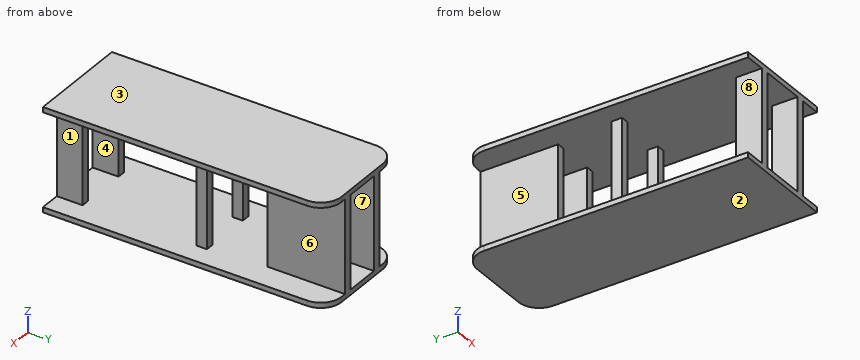
```python
from build123d import *

# Parameters (mm, degrees)
SKETCH_1_W      = 200
SKETCH_1_H      = 550
EXTRUDE_2_DEPTH = 10
FILLET_2_R      = 40
SKETCH_2_W      = 16
SKETCH_2_H      = 50
SKETCH_2_H_2    = 20
SKETCH_2_H_3    = 150
EXTRUDE_4_DEPTH = 90
SKETCH_3_W      = 200
SKETCH_3_H      = 550
EXTRUDE_5_DEPTH = 10
FILLET_5_R      = 40


with BuildPart() as part:
    # 스케치1 → 보스-돌출2 (new body)
    with BuildSketch(Plane.XY):
        with Locations((100, 275)):
            Rectangle(SKETCH_1_W, SKETCH_1_H)
    extrude(amount=EXTRUDE_2_DEPTH)

    # 필렛2
    fillet_2_edges = [part.edges().sort_by_distance(p)[0] for p in [
        (0, 550, 5),
        (200, 550, 5),
    ]]
    fillet(fillet_2_edges, radius=FILLET_2_R)

    # 스케치2 → 보스-돌출4 (add)
    with BuildSketch(Plane.XY.offset(10)):
        with Locations((152, 25)):
            Rectangle(SKETCH_2_W, SKETCH_2_H)
        with Locations((152, 280)):
            Rectangle(SKETCH_2_W, SKETCH_2_H_2)
        with Locations((142, 475)):
            Rectangle(SKETCH_2_W, SKETCH_2_H_3)
        with Locations((48, 25)):
            Rectangle(SKETCH_2_W, SKETCH_2_H)
        with Locations((48, 280)):
            Rectangle(SKETCH_2_W, SKETCH_2_H_2)
        with Locations((58, 475)):
            Rectangle(SKETCH_2_W, SKETCH_2_H_3)
    extrude_4 = extrude(amount=EXTRUDE_4_DEPTH)

    # 대칭 복사26: 보스-돌출4 across plane
    add(extrude_4.mirror(Plane(origin=(0, 0, 100), x_dir=(1, 0, 0), z_dir=(0, 0, -1))))

    # 스케치3 → 보스-돌출5 (add)
    with BuildSketch(Plane.XY.offset(190)):
        with Locations((100, 275)):
            Rectangle(SKETCH_3_W, SKETCH_3_H)
    extrude(amount=EXTRUDE_5_DEPTH)

    # 필렛5
    fillet_5_edges = [part.edges().sort_by_distance(p)[0] for p in [
        (0, 550, 195),
        (200, 550, 195),
    ]]
    fillet(fillet_5_edges, radius=FILLET_5_R)


solid = part.part
```
Geometry: final body of the model. Coordinates: model frame, mm. Face numbers are marked on the shaded views. A direction names the side the tool comes from. Round coordinates to 2 decimals unless told otherwise and drop trailing zeros. Write each loop counter-clockwise with the first axis right and the second up, starting at its lowest first coordinate (ties: lowest second). Pieces come first, ordered by that corner, then holes.
Item 1: Pin query (flat end, axial travel): P1, Ø1.5, axis at y = 289.5, z = 164, coming from the -X side; P2, Ø8, axis at x = 138.5, z = 102.5, coming from the -Y side; P3, Ø5, axis at x = 155.5, z = 102.5, coming from the +Y side. Return the tip coordinate at first contact, or that it passes through.
Item 2: Section query C-C (y = 90). Return loops of the section in (x, z).
Item 3: Section query A-A (z = 27). Return loops of the section in (x, y).
Item 4: Mould query, pull axis Z, two halves, no side actions, for the marked faces 1, 2 and 3. Classes: +Z half, -Z half, draft (parallel to the pull), parting line (faces both ways), or undercut.
Item 5: Set-up query: the marked faces 4, 5, 6, 7 and 8. Return all of +Z, -Z, +X, -X, +Y, -Y with unobstructed straight access to the full face (end or side cutting, diameter ignored); none if empty.
Item 6: Section query B-B (x = 155). Return loops of the section in (y, z), plus the area to 3 significant figures.
Item 7: Material intervals for L1, parallel to Y at x = 52.5, z = 152.5; L2, parallel to Z at x = 94, y = 479; L3, parallel to X at y = 288.5, z = 12, sorted ascending.
Item 8: Section query D-D (x = 115.5). Return loops of the section in (y, z).
Completed:
1. P1: stops at x = 40
1. P2: stops at y = 400
1. P3: stops at y = 290
2. outline: (0, 0) - (200, 0) - (200, 10) - (0, 10) - close; (0, 190) - (200, 190) - (200, 200) - (0, 200) - close
3. outline: (40, 0) - (56, 0) - (56, 50) - (40, 50) - close; (40, 270) - (56, 270) - (56, 290) - (40, 290) - close; (50, 400) - (66, 400) - (66, 550) - (50, 550) - close; (134, 400) - (150, 400) - (150, 550) - (134, 550) - close; (144, 0) - (160, 0) - (160, 50) - (144, 50) - close; (144, 270) - (160, 270) - (160, 290) - (144, 290) - close
4. face 1: undercut
4. face 2: -Z half
4. face 3: +Z half
5. face 4: -Y
5. face 5: -X, +Y
5. face 6: +X, +Y
5. face 7: +Y, -Y
5. face 8: -X, +Y, -Y
6. outline: (0, 0) - (550, 0) - (550, 10) - (290, 10) - (290, 190) - (550, 190) - (550, 200) - (0, 200) - close; hole (50, 10) - (270, 10) - (270, 190) - (50, 190) - close
6. area: 23,600 mm2
7. L1: y = 0 to 50, 270 to 290, 400 to 550
7. L2: z = 0 to 10, 190 to 200
7. L3: x = 40 to 56, 144 to 160
8. outline: (0, 0) - (550, 0) - (550, 10) - (0, 10) - close; (0, 190) - (550, 190) - (550, 200) - (0, 200) - close
